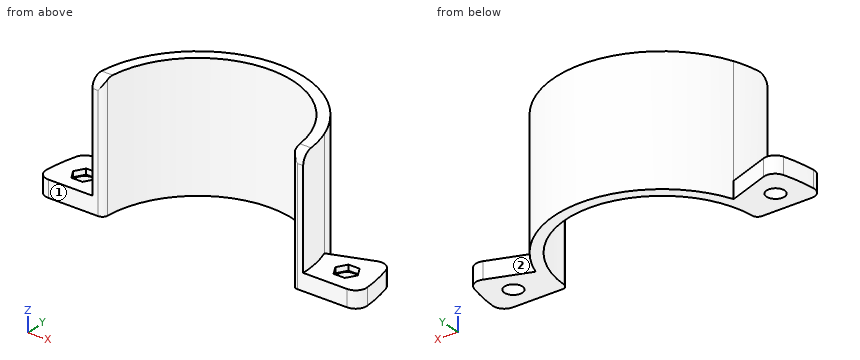
```python
from build123d import *
from OCP.BRepFilletAPI import BRepFilletAPI_MakeFillet

# Parameters (mm, degrees)
SKETCH2_R             = 1.6
BOSS_EXTRUDE1_DEPTH   = 3
BOSS_EXTRUDE1_2_DEPTH = 3
BOSS_EXTRUDE2_DEPTH   = 22.5
FILLET1_R1            = 2
FILLET1_R2            = 1
CUT_EXTRUDE2_DEPTH    = 1


with BuildPart() as part:
    # Sketch2 → Boss-Extrude1 (new body)
    with BuildSketch(Plane.XY):
        with BuildLine():
            ThreePointArc((-19, 0), (-18.711347307, 3.299315376), (-17.854159795, 6.498382723))
            Line((-17.854159795, 6.498382723), (-27.251086003, 9.918584156))
            ThreePointArc((-27.251086003, 9.918584156), (-28.559424837, 5.035797152), (-29, 0))
            Line((-29, 0), (-19, 0))
        make_face()
        with Locations((-23.635386072, 4.167556264)):
            Circle(SKETCH2_R, mode=Mode.SUBTRACT)
    extrude(amount=BOSS_EXTRUDE1_DEPTH)



with BuildPart() as body_2:
    # Sketch2 → Boss-Extrude1 2 (new body)
    with BuildSketch(Plane.XY):
        with BuildLine():
            ThreePointArc((17.854159795, 6.498382723), (18.711347307, 3.299315376), (19, 0))
            Line((19, 0), (29, 0))
            ThreePointArc((29, 0), (28.559424837, 5.035797152), (27.251086003, 9.918584156))
            Line((27.251086003, 9.918584156), (17.854159795, 6.498382723))
        make_face()
        with Locations((23.635386072, 4.167556264)):
            Circle(SKETCH2_R, mode=Mode.SUBTRACT)
    extrude(amount=BOSS_EXTRUDE1_2_DEPTH)


with BuildPart() as part_1:
    add(part.part)

    add(body_2.part)  # Boss-Extrude2 merges body 2
    # Sketch2<3> → Boss-Extrude2 (add)
    with BuildSketch(Plane.XY):
        with BuildLine():
            Line((-19, 0), (-17, 0))
            ThreePointArc((-17, 0), (0, 17), (17, 0))
            Line((17, 0), (19, 0))
            ThreePointArc((19, 0), (18.711347307, 3.299315376), (17.854159795, 6.498382723))
            ThreePointArc((17.854159795, 6.498382723), (0, 19), (-17.854159795, 6.498382723))
            ThreePointArc((-17.854159795, 6.498382723), (-18.711347307, 3.299315376), (-19, 0))
        make_face()
    extrude(amount=BOSS_EXTRUDE2_DEPTH)

    # Fillet1: one fillet with a radius per group of edges: ONE call of the kernel's fillet builder (fillet() takes one radius for all edges)
    fillet1_edges_1 = [part_1.edges().sort_by_distance(p)[0] for p in [
        (-29, 0, 1.5),
        (-27.251086003, 9.918584156, 1.5),
        (-18, 0, 22.5),
        (18, 0, 22.5),
        (29, 0, 1.5),
        (27.251086003, 9.918584156, 1.5),
    ]]
    fillet1_edges_2 = [part_1.edges().sort_by_distance(p)[0] for p in [
        (-17, 0, 11.25),
        (17, 0, 11.25),
    ]]
    fillet1 = BRepFilletAPI_MakeFillet(part_1.part.solid().wrapped)
    for e in fillet1_edges_1:
        fillet1.Add(FILLET1_R1, e.wrapped)
    for e in fillet1_edges_2:
        fillet1.Add(FILLET1_R2, e.wrapped)
    add(Compound.cast(fillet1.Shape()), mode=Mode.REPLACE)

    # Sketch4 → Cut-Extrude2 (cut)
    with BuildSketch(Plane.XY.offset(3)):
        Polygon((-21.61466013, 4.167556264), (-22.625023101, 5.917556264), (-24.645749043, 5.917556264), (-25.656112014, 4.167556264), (-24.645749043, 2.417556264), (-22.625023101, 2.417556264), align=None)
        Polygon((25.656112014, 4.167556264), (24.645749043, 5.917556264), (22.625023101, 5.917556264), (21.61466013, 4.167556264), (22.625023101, 2.417556264), (24.645749043, 2.417556264), align=None)
    extrude(amount=-CUT_EXTRUDE2_DEPTH, mode=Mode.SUBTRACT)


solid = part_1.part
```
For this review, take the finished solid that the model builds, in its own axes (mm). Face numbers are marked on the shaded views. A direction names the side the tool comes from. Give positions to 0.01 mm unless a question says otherwise; leave off trailing zeros. Write each loop counter-clockwise with the first axis right and the second up, starting at its lowest first coordinate (ties: lowest second). Pieces come first, ordered by that corner, then holes.
Item 1: Insertion check: P1, Ø2, axis at x = -9.5, z = 13.5, coming from the +Y side; P2, Ø7.5, axis at x = -25, y = 4, coming from the +Z side; P3, Ø1, axis at x = 15, z = 3.5, coming from the +Y side. Each pin has a flat end and moves straight along its axis. Give the tip position at first contact, or say it passes through.
Item 2: Take a section at D-D (x = 0). Give the boundary of the cut face in (y, z), and give its area (3 significant figures).
Item 3: Wall thickness on probe 1 along X at (y, z) = (2, 15.5); probe 2 along X at (y, z) = (7.25, 3.5); probe 3 along Z at (x, y) = (20, 3.25): over which ranges is each line inside the solid? List them lowest first.
Item 4: Take a section at B-B (y = 11). Give the boundary of the cut face in (x, z).
Item 5: Machinability: for the marked faces 1 and 2, which of the approach directions +Z, -Z, +X, -X, +Y, -Y give a long, thin tool a straight path to every point of the face, cutting with its end or side? Answer none if there is none.
Item 6: Take a section at A-A (x = 24). Give the boundary of the cut face in (y, z), and give its area (3 significant figures).
Established:
1. P1: stops at y = 16.99
1. P2: stops at z = 3
1. P3: stops at y = 12.28
2. outline: (17, 0) - (19, 0) - (19, 22.5) - (17, 22.5) - close
2. area: 45.0 mm2
3. probe 1: x = -18.89 to -16.88, 16.88 to 18.89
3. probe 2: x = -17.56 to -15.38, 15.38 to 17.56
3. probe 3: z = 0 to 3
4. outline: (-15.49, 0) - (-12.96, 0) - (-12.96, 22.5) - (-15.49, 22.5) - close; (12.96, 0) - (15.49, 0) - (15.49, 22.5) - (12.96, 22.5) - close
5. face 1: +Z, -Z, +X, -X, -Y
5. face 2: +Z, -Z, +Y
6. outline: (0, 0) - (2.61, 0) - (2.61, 2) - (2.42, 2) - (2.42, 3) - (0, 3) - close; (5.73, 0) - (8.74, 0) - (8.74, 3) - (5.92, 3) - (5.92, 2) - (5.73, 2) - close
6. area: 16.5 mm2
